from build123d import *

# Parameters (mm, degrees)
SKETCH2_W           = 6.35
SKETCH2_H           = 24.593444248
SKETCH3_W           = 6.35
SKETCH3_H           = 24.593444248
BOSS_EXTRUDE1_DEPTH = 15.24
SKETCH4_R           = 6.35
CUT_EXTRUDE1_DEPTH  = 30.655247945


with BuildPart() as part:
    # Sketch2 → Loft1 section 0
    with BuildSketch(Plane.XY.offset(6.35)):
        Rectangle(SKETCH2_W, SKETCH2_H)
    # Sketch1 for Loft1 → Loft1 section 1
    with BuildSketch(Plane.XY):
        with BuildLine():
            # circular arc as an exact rational Bezier (weights 1, cos(half-angle), 1)
            Bezier((-3.175, 12.296722124), (0, 13.116503599), (3.175, 12.296722124), weights=[1, 0.968245837, 1])
            Bezier((3.175, 12.296722124), (50.800000002, 0), (3.175, -12.296722124), weights=[1, 0.25, 1])
            Bezier((3.175, -12.296722124), (0, -13.116503599), (-3.175, -12.296722124), weights=[1, 0.968245837, 1])
            Bezier((-3.175, -12.296722124), (-50.800000002, 0), (-3.175, 12.296722124), weights=[1, 0.25, 1])
        make_face()
    loft()

    # Sketch3 → Boss-Extrude1 (add)
    with BuildSketch(Plane.XY.offset(6.35)):
        Rectangle(SKETCH3_W, SKETCH3_H)
    extrude(amount=BOSS_EXTRUDE1_DEPTH)

    # Sketch4 → Cut-Extrude1 (cut, through all)
    with BuildSketch(Plane(origin=(3.175, 0, 0), x_dir=(0, 0, -1), z_dir=(1, 0, 0))):
        with Locations((-12.7, 1.010428855)):
            Circle(SKETCH4_R)
    extrude(amount=-CUT_EXTRUDE1_DEPTH, mode=Mode.SUBTRACT)


solid = part.part
Verification items for the finished model (mm, model axes). A direction names the side the tool comes from. Round coordinates to 2 decimals unless told otherwise and drop trailing zeros. Write each loop counter-clockwise with the first axis right and the second up, starting at its lowest first coordinate (ties: lowest second). Pieces come first, ordered by that corner, then holes.
(1) Mould release check, pull along Y, two halves, no side actions. Record for faces 1 (the flat face through (0, -12.297, 14)), 2 (the cylindrical face through (0.044, -1.422, 6.834)), 3 (the flat face through (0, 12.297, 14)), 4 (the flat face through (3.175, -6, 14)): pulls with the +Y half, pulls with the -Y half, needs draft (parallel to the pull), parting line crosses it, or undercut.
Returned:
face 1: pulls with the -Y half
face 2: undercut
face 3: pulls with the +Y half
face 4: needs draft
(2) Access from +Z, -Z, +X, -X, +Y, -Y to the whole of each face (thin tool, end or side, straight path). Record for faces 5 (the flat face through (-3.175, -6, 14)), 6 (the flat face through (1, 2, 0)).
Returned:
face 5: +Z, -X, +Y, -Y
face 6: -Z, +X, -X, +Y, -Y
(3) Section check A-A (z = 12.7). Enter the section's corners in (x, y) (3 decimals), plus the area to 3 significant figures.
Returned:
outline: (-3.175, -12.297) - (3.175, -12.297) - (3.175, -5.34) - (-3.175, -5.34) - close; (-3.175, 7.36) - (3.175, 7.36) - (3.175, 12.297) - (-3.175, 12.297) - close
area: 75.5 mm2
(4) Depth check by flat-ended pin: pin 1 Ø8 at (x, z) = (6.5, 16) entering from +Y; pin 2 Ø3 at (x, z) = (1, 12) entering from -Y. Enter the tip coordinate at first touch or a pass-through.
Returned:
pin 1: stops at y = 12.3
pin 2: stops at y = -12.3
(5) Material ranges on line 1 (Y direction, x = 0, z = 12.7); line 2 (X direction, y = 11, z = 16.75) (3 decimals); line 3 (Y direction, x = -2.5, z = 16.5), recorded low to high.
Returned:
line 1: y = -12.3 to -5.34, 7.36 to 12.3
line 2: x = -3.175 to 3.175
line 3: y = -12.3 to -4.08, 6.1 to 12.3
